```python
from build123d import *

# Parameters (mm, degrees)
CHAMFER3_SIZE  = 0.5
CHAMFER3_SIZE2 = 0.524090046


with BuildPart() as part:
    # Sketch4 → Revolve1 (revolve)
    with BuildSketch(Plane.XY, mode=Mode.PRIVATE) as revolve1_sk:
        Polygon((0, 0), (0, 20), (0, 25), (1.25, 25), (1.25, 20), (2.5, 20), (3.175, 5), (3.175, 0), align=None)
    revolve(revolve1_sk.sketch.rotate(Axis((0, 0, 0), (0, 1, 0)), 90), axis=Axis((0, 0, 0), (0, 1, 0)))

    # Chamfer3
    chamfer3_edges = [part.edges().sort_by_distance(p)[0] for p in [
        (0, 20, 2.5),
    ]]
    chamfer3_side = [part.faces().sort_by_distance(p)[0] for p in [
        (0, 20, 1.320710678),
    ]]
    chamfer(chamfer3_edges, length=CHAMFER3_SIZE, length2=CHAMFER3_SIZE2, reference=chamfer3_side[0])


solid = part.part
```
Verification items for the finished model (mm, model axes). A direction names the side the tool comes from. Round coordinates to 2 decimals unless told otherwise and drop trailing zeros. Loops run counter-clockwise (first coordinate to the right, second up) from the corner with the lowest first, then second, coordinate; pieces in that order, holes last. Notation, with made-up numbers: (20.25, -14) -> (48.25, -14) arc R11 ccw to (48.25, 3) -> close; hole circle Ø11 at (79, 1.25). An arc over 180 degrees is marked (long way). Answer as a JSON object with one key per item and string values.
Q1. Go/stop test with flat-tipped pins: P1, Ø3, axis at y = 3.5, z = -2, coming from the +X side; P2, Ø3, axis at y = 15.5, z = 0.5, coming from the -X side; P3, Ø2, axis at y = 14, z = 2, coming from the +X side. Record where each tip stops, or that it passes through.
Data:
{"P1": "stops at x = 3.14", "P2": "stops at x = -2.77", "P3": "stops at x = 2.59"}
Q2. Section check B-B (x = 0). Record the boundary of the cut face in (y, z) (3 decimals), then the cut area to 3 significant figures.
Data:
{"outline": "(0, -3.175) -> (5, -3.175) -> (19.476, -2.524) -> (20, -2) -> (20, -1.25) -> (25, -1.25) -> (25, 1.25) -> (20, 1.25) -> (20, 2) -> (19.476, 2.524) -> (5, 3.175) -> (0, 3.175) -> close", "area": "129 mm2"}
Q3. Section check A-A (z = 0). Record the boundary of the cut face in (x, y) (3 decimals), then the cut area to 3 significant figures.
Data:
{"outline": "(-3.175, 0) -> (3.175, 0) -> (3.175, 5) -> (2.524, 19.476) -> (2, 20) -> (1.25, 20) -> (1.25, 25) -> (-1.25, 25) -> (-1.25, 20) -> (-2, 20) -> (-2.524, 19.476) -> (-3.175, 5) -> close", "area": "129 mm2"}
Q4. Section check C-C (y = 4.25). Record the boundary of the cut face in (x, z) (3 decimals), then the cut area to 3 significant figures.
Data:
{"outline": "circle Ø6.35 at (0, 0)", "area": "31.7 mm2"}
Q5. Scan lines: line 1 (X direction, y = 19.5, z = -1.5); line 2 (Y direction, x = 0.25, z = 1.75); line 3 (X direction, y = 6, z = -1.25). Record each from-to range of solid material in increasing order. Write a range as from..to.
Data:
{"line 1": "x = -2..2", "line 2": "y = 0..20", "line 3": "x = -2.87..2.87"}
Q6. Access from +Z, -Z, +X, -X, +Y, -Y to the whole of each face (thin tool, end or side, straight path). Record for faces 1 (the flat face through (-1, 20, 1)), 2 (the flat face through (0, 0, 0)).
Data:
{"face 1": "+Y", "face 2": "+Z, -Z, +X, -X, -Y"}
Q7. Section check D-D (y = 10). Record the boundary of the cut face in (x, z), then the cut area to 3 significant figures.
Data:
{"outline": "circle Ø5.9 at (0, 0)", "area": "27.3 mm2"}
